Geometry check sheet. Reference: the model listing, model coordinates, mm. A direction names the side the tool comes from. Give positions to 0.01 mm unless a question says otherwise; leave off trailing zeros. Loops run counter-clockwise (first coordinate to the right, second up) from the corner with the lowest first, then second, coordinate; pieces in that order, holes last. Notation, with made-up numbers: (-8.75, 0.25) - (17.25, 0.25) arc R30 cw to (17.25, 26.25) - close; hole circle Ø5 at (41.5, 29.25). An arc over 180 degrees is marked (long way). Write item = value, one per line. Start each with the question number.
from build123d import *

# Parameters (mm, degrees)
SKETCH029_W   = 8.5
SKETCH029_H   = 44
PAD002_DEPTH  = 20
SKETCH023_R   = 1.5
HOLE004_DEPTH = 4
SKETCH032_R   = 1.5
HOLE006_DEPTH = 4
SKETCH034_W   = 44
SKETCH034_H   = 6
POCKET_DEPTH  = 7


with BuildPart() as part:
    # Sketch029 → Pad002 (new body)
    with BuildSketch(Plane.XY):
        with Locations((-4.25, 22)):
            Rectangle(SKETCH029_W, SKETCH029_H)
    extrude(amount=PAD002_DEPTH)

    # Sketch023 → Hole004 (cut)
    with BuildSketch(Plane.XY):
        with Locations((-4.250802, 4.5)):
            Circle(SKETCH023_R)
        with Locations((-4.25, 39.500714)):
            Circle(SKETCH023_R)
        with Locations((-4.254534, 22)):
            Circle(SKETCH023_R)
        with Locations((-4.25, 4.5)):
            Circle(SKETCH023_R)
    extrude(amount=HOLE004_DEPTH, mode=Mode.SUBTRACT)

    # Sketch032 (on Face5 of Hole004) → Hole006 (cut)
    with BuildSketch(Plane.XY.offset(20)):
        with Locations((-4.250802, 4.5)):
            Circle(SKETCH032_R)
        with Locations((-4.25, 39.499999)):
            Circle(SKETCH032_R)
        with Locations((-4.254534, 22)):
            Circle(SKETCH032_R)
        with Locations((-4.25, 4.5)):
            Circle(SKETCH032_R)
    extrude(amount=-HOLE006_DEPTH, mode=Mode.SUBTRACT)

    # Sketch034 (on Face3 of Hole006) → Pocket (cut)
    with BuildSketch(Plane(origin=(-8.5, 0, 0), x_dir=(0, -1, 0), z_dir=(-1, 0, 0))):
        with Locations((-22, 5)):
            Rectangle(SKETCH034_W, SKETCH034_H)
    extrude(amount=-POCKET_DEPTH, mode=Mode.SUBTRACT)


solid = part.part
1) Cross-section at D-D on z = 5.5. Enter the section's corners in (x, y).
2) Release check for a two-part mould opening along Y. For faces 4 (the face through (-8.5, 22, 1)), 5 (the face through (-4.445, 40.987, 18.028)), 6 (the face through (-4, 44, 12)), 7 (the face through (-4, 40, 16)) record: pulls with the +Y half, pulls with the -Y half, needs draft (parallel to the pull), parting line crosses it, or undercut.
3) Gauge pin test, flat ends, axial feed: P1, Ø3, axis at y = 23, z = 4, coming from the -X side; P2, Ø1.5, axis at x = -3.5, y = 5, coming from the +Z side; P3, Ø2.5, axis at x = -4.25, y = 39.5, coming from the -Z side; P4, Ø2.5, axis at x = -4.25, y = 39.5, coming from the +Z side. Record the tip position at first contact, or that the pin passes through.
4) Cross-section at C-C on y = 9.5. Enter the section's corners in (x, z), and give its area (3 significant figures).
5) Tool access check on faces 1 (the face through (-5.44, 38.59, 0.99)), 2 (the face through (-4.45, 23.487, 18.028)), 3 (the face through (-1.5, 22, 5)). Record the directions out of +Z, -Z, +X, -X, +Y, -Y that give a thin tool (end or side, any length) a straight path to the whole face; none if there is none.
6) Material ranges on line 1 along Y through (x, z) = (-4.25, 1.2); line 2 along Z through (x, y) = (-5.25, 17.5); line 3 along X through (y, z) = (22, 1.2), recorded low to high.
7) Cross-section at A-A on x = -2. Enter the section's corners in (y, z).
8) Cross-section at B-B on y = 4.5. Enter the section's corners in (x, z), and give its area (3 significant figures).
Checked values:
q1.outline = (-1.5, 0) - (0, 0) - (0, 44) - (-1.5, 44) - close
q2.face_4 = needs draft
q2.face_5 = undercut
q2.face_6 = pulls with the +Y half
q2.face_7 = undercut
q3.P1 = -1.5
q3.P2 = 20
q3.P3 = 8
q3.P4 = 16
q4.outline = (-8.5, 0) - (0, 0) - (0, 20) - (-8.5, 20) - (-8.5, 8) - (-1.5, 8) - (-1.5, 2) - (-8.5, 2) - close
q4.area = 128 mm²
q5.face_1 = -Z
q5.face_2 = +Z
q5.face_3 = -X, +Y, -Y
q6.line_1 = 0 to 3, 6 to 20.5, 23.5 to 38, 41 to 44
q6.line_2 = 0 to 2, 8 to 20
q6.line_3 = -8.5 to -5.75, -2.75 to 0
q7.outline = (0, 0) - (44, 0) - (44, 2) - (0, 2) - close; (0, 8) - (44, 8) - (44, 20) - (0, 20) - close
q8.outline = (-8.5, 0) - (-5.75, 0) - (-5.75, 2) - (-8.5, 2) - close; (-8.5, 8) - (-1.5, 8) - (-1.5, 2) - (-2.75, 2) - (-2.75, 0) - (0, 0) - (0, 20) - (-2.75, 20) - (-2.75, 16) - (-5.75, 16) - (-5.75, 20) - (-8.5, 20) - close
q8.area = 110 mm²
